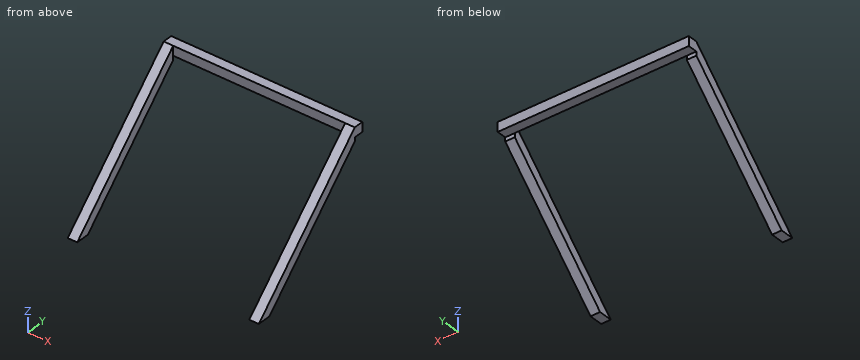
from build123d import *

# Parameters (mm, degrees)
F2_DEPTH = 25.4
F3_W     = 25.4
F3_H     = 25.4
F4_DEPTH = 254


with BuildPart() as f2:
    # F1 (on offset) → F2 (new body)
    with BuildSketch(Plane.YZ.offset(228.6)):
        Polygon((323.28922, 323.28922), (0, 0), (35.921024, 0), (323.28922, 287.368196), align=None)
    extrude(amount=F2_DEPTH)

    # F3 (on Right) → F4 (join, through all)
    with BuildSketch(Plane.YZ):
        with Locations((335.98922, 310.58922)):
            Rectangle(F3_W, F3_H)
    extrude(amount=F4_DEPTH)

    # F5: F2 across plane


with BuildPart() as f2_1:
    add(f2.part)
    add(f2.part.mirror(Plane.YZ))


solid = f2_1.part
Geometry check sheet. Reference: the model listing, model coordinates, mm. Round coordinates to 2 decimals unless told otherwise and drop trailing zeros. Write each loop counter-clockwise with the first axis right and the second up, starting at its lowest first coordinate (ties: lowest second). Pieces come first, ordered by that corner, then holes.
Item 1: Section check A-A (y = 48). Record the boundary of the cut face in (x, z), plus the area to 3 significant figures.
Determined:
outline: (-254, 12.08) - (-228.6, 12.08) - (-228.6, 48) - (-254, 48) - close; (228.6, 12.08) - (254, 12.08) - (254, 48) - (228.6, 48) - close
area: 1,820 mm2
Item 2: Go/stop test with flat-tipped pins: pin 1 Ø8.5 at (x, z) = (242, 290) entering from +Y; pin 2 Ø20.5 at (x, y) = (-78.5, 342) entering from -Z; pin 3 Ø7.5 at (x, z) = (4.5, 308.5) entering from -Y. Record where each tip stops, or that it passes through.
Determined:
pin 1: stops at y = 323.29
pin 2: stops at z = 297.89
pin 3: stops at y = 323.29
Item 3: Section check C-C (x = 76). Record the boundary of the cut face in (y, z), plus the area to 3 significant figures.
Determined:
outline: (323.29, 297.89) - (348.69, 297.89) - (348.69, 323.29) - (323.29, 323.29) - close
area: 645 mm2
Item 4: Section check B-B (z = 135). Record the boundary of the cut face in (x, y), plus the area to 3 significant figures.
Determined:
outline: (-254, 135) - (-228.6, 135) - (-228.6, 170.92) - (-254, 170.92) - close; (228.6, 135) - (254, 135) - (254, 170.92) - (228.6, 170.92) - close
area: 1,820 mm2
Item 5: Material ranges on line 1 along X through (y, z) = (292, 288.5); line 2 along Y through (x, z) = (79, 298.5), recorded low to high.
Determined:
line 1: x = -254 to -228.6, 228.6 to 254
line 2: y = 323.29 to 348.69
